from build123d import *

# Parameters (mm, degrees)
F0_R     = 11.1125
F1_DEPTH = 7
F2_W     = 6.35
F2_H     = 6.35
F3_DEPTH = 7


with BuildPart() as f1:
    # F0 (on Top) → F1 (new body)
    with BuildSketch(Plane.XY):
        with BuildLine():
            ThreePointArc((-50.8, 0), (-46.15032, -11.22532), (-34.925, -15.875))
            Line((-34.925, -15.875), (-26.135577, -15.875))
            Line((-26.135577, -15.875), (26.135577, -15.875))
            Line((26.135577, -15.875), (34.925, -15.875))
            ThreePointArc((34.925, -15.875), (46.15032, -11.22532), (50.8, 0))
            ThreePointArc((50.8, 0), (46.15032, 11.22532), (34.925, 15.875))
            Line((34.925, 15.875), (26.135577, 15.875))
            Line((26.135577, 15.875), (-26.135577, 15.875))
            ThreePointArc((-26.135577, 15.875), (-34.22483, 20.309354), (-34.837518, 29.513925))
            ThreePointArc((-34.837518, 29.513925), (-46.553742, 16.777013), (-50.8, 0))
        make_face()
        with Locations((-34.925, 0)):
            Circle(F0_R, mode=Mode.SUBTRACT)
        Circle(F0_R, mode=Mode.SUBTRACT)
        with Locations((34.925, 0)):
            Circle(F0_R, mode=Mode.SUBTRACT)
        with BuildLine():
            Line((-26.135577, -15.875), (-34.925, -15.875))
            ThreePointArc((-34.925, -15.875), (-46.15032, -11.22532), (-50.8, 0))
            ThreePointArc((-50.8, 0), (-46.553742, -16.777013), (-34.837518, -29.513925))
            ThreePointArc((-34.837518, -29.513925), (-34.22483, -20.309354), (-26.135577, -15.875))
        make_face()
        with BuildLine():
            Line((34.925, -15.875), (26.135577, -15.875))
            ThreePointArc((26.135577, -15.875), (34.22483, -20.309354), (34.837518, -29.513925))
            ThreePointArc((34.837518, -29.513925), (46.553742, -16.777013), (50.8, 0))
            ThreePointArc((50.8, 0), (46.15032, -11.22532), (34.925, -15.875))
        make_face()
        with BuildLine():
            ThreePointArc((34.925, 15.875), (46.15032, 11.22532), (50.8, 0))
            ThreePointArc((50.8, 0), (46.553742, 16.777013), (34.837518, 29.513925))
            ThreePointArc((34.837518, 29.513925), (34.22483, 20.309354), (26.135577, 15.875))
            Line((26.135577, 15.875), (34.925, 15.875))
        make_face()
    extrude(amount=F1_DEPTH)

    # F2 (on face) → F3 (cut, through all)
    with BuildSketch(Plane.XY.offset(7)):
        with Locations((17.4625, 0)):
            Rectangle(F2_W, F2_H)
        with Locations((-17.4625, 0)):
            Rectangle(F2_W, F2_H)
    extrude(amount=-F3_DEPTH, mode=Mode.SUBTRACT)


solid = f1.part
Source: CAD feature listing. Evaluate the final solid. Frame: model axes, mm. A direction names the side the tool comes from. Coordinates: 2 decimals unless noted, no trailing zeros. Loops run counter-clockwise (first coordinate to the right, second up) from the corner with the lowest first, then second, coordinate; pieces in that order, holes last. Notation, with made-up numbers: (-26.75, 47.25) - (24.25, 47.25) arc R21 cw to (24.25, 73.25) - close; hole circle Ø11 at (82.25, 72.5). An arc over 180 degrees is marked (long way). One line per item, written item: value. Start each with the question number.
1. Section C-C (y = -7). Return the cut outline in (x, z), and give its area (3 significant figures).
2. Ray query, L1, parallel to X at y = 8.5, z = 6.5; L2, parallel to Y at x = 0, z = 4.75 (1 decimal); L3, parallel to X at y = -5.5, z = 6.5. Return the intervals inside material, ascending.
3. Contact query for flat-ended pins moving along their axis: P1, Ø3, axis at x = -18, z = 3, coming from the -Y side (3 decimals); P2, Ø3.5, axis at x = 5, z = 3, coming from the +Y side (3 decimals); P3, Ø1.5, axis at y = -19.5, z = 3, coming from the -X side. Output: stop coordinate, or through.
4. Section D-D (y = 25). Return the cut outline in (x, z), and give its area (3 significant figures).
5. Section A-A (x = 16). Return the cut outline in (y, z) (3 decimals), and give its area (3 significant figures).
6. Section B-B (z = 1.5). Return the cut outline in (x, y) (1 decimal).
7. Mould query, pull axis X, two halves, no side actions, for faces 4 (the flat face through (-12, 0, 0)), 5 (the cylindrical face through (34.296, 20.423, 3.451)). Classes: pulls with the +X half, pulls with the -X half, needs draft (parallel to the pull), parting line crosses it, or undercut.
8. Set-up query: faces 1 (the flat face through (0, 15.875, 3)), 2 (the flat face through (-12, 0, 7)), 3 (the flat face through (17, -3.175, 4)). Return all of +Z, -Z, +X, -X, +Y, -Y with unobstructed straight access to the full face (end or side cutting, diameter ignored); none if empty.
Verdict:
1. outline: (-50.1, 0) - (-43.56, 0) - (-43.56, 7) - (-50.1, 7) - close; (-26.29, 0) - (-8.63, 0) - (-8.63, 7) - (-26.29, 7) - close; (8.63, 0) - (26.29, 0) - (26.29, 7) - (8.63, 7) - close; (43.56, 0) - (50.1, 0) - (50.1, 7) - (43.56, 7) - close
1. area: 339 mm2
2. L1: x = -49.76 to -42.08, -27.77 to -7.16, 7.16 to 27.77, 42.08 to 49.76
2. L2: y = -15.9 to -11.1, 11.1 to 15.9
2. L3: x = -50.37 to -44.58, -25.27 to -9.66, 9.66 to 25.27, 44.58 to 50.37
3. P1: stops at y = -15.875
3. P2: stops at y = 15.875
3. P3: stops at x = -45.4
4. outline: (-40.41, 0) - (-35.72, 0) - (-35.72, 7) - (-40.41, 7) - close; (35.72, 0) - (40.41, 0) - (40.41, 7) - (35.72, 7) - close
4. area: 65.6 mm2
5. outline: (-15.875, 0) - (-3.175, 0) - (-3.175, 7) - (-15.875, 7) - close; (3.175, 0) - (15.875, 0) - (15.875, 7) - (3.175, 7) - close
5. area: 178 mm2
6. outline: (-50.8, 0) arc R35.3 ccw to (-34.8, -29.5) arc R9.6 cw to (-26.1, -15.9) - (26.1, -15.9) arc R9.6 cw to (34.8, -29.5) arc R35.3 ccw to (50.8, 0) arc R35.3 ccw to (34.8, 29.5) arc R9.6 cw to (26.1, 15.9) - (-26.1, 15.9) arc R9.6 cw to (-34.8, 29.5) arc R35.3 ccw to start; hole circle Ø22.2 at (-34.9, 0); hole (-20.6, -3.2) - (-14.3, -3.2) - (-14.3, 3.2) - (-20.6, 3.2) - close; hole circle Ø22.2 at (0, 0); hole (14.3, -3.2) - (20.6, -3.2) - (20.6, 3.2) - (14.3, 3.2) - close; hole circle Ø22.2 at (34.9, 0)
7. face 4: needs draft
7. face 5: undercut
8. face 1: +Z, -Z, +Y
8. face 2: +Z, +X, -X, +Y, -Y
8. face 3: +Z, -Z
